Build history of the part. All positions in model axes, mm. A direction names the side the tool comes from. Give positions to 0.01 mm unless a question says otherwise; leave off trailing zeros. Write each loop counter-clockwise with the first axis right and the second up, starting at its lowest first coordinate (ties: lowest second). Pieces come first, ordered by that corner, then holes. Notation, with made-up numbers: (-6, 9.25) -> (7, 9.25) arc R18 ccw to (7, 32.25) -> close; hole circle Ø2 at (69.5, 9). An arc over 180 degrees is marked (long way). Put each result on its own line as item: value. Start each with the question number.
Item 1: Slice it at C-C, the plane y = 13. List the corners of the cut face in (x, z), plus the area to 3 significant figures.
Item 2: Tool access for faces 1 (the flat face through (38, 47, 0.5)), 2 (the flat face through (75.2, 12, 1)), 3 (the flat face through (-3, 35, 1)), 4 (the flat face through (75.2, 47, 1)), 5 (the flat face through (-4, 25, 1)): list every direction of +Z, -Z, +X, -X, +Y, -Y with a clear straight run to the whole face (end or side of a thin tool).
Item 3: Slice it at A-A, the plane y = 30. List the corners of the cut face in (x, z).
Item 4: Slice it at D-D, the plane y = 38.5. List the corners of the cut face in (x, z), plus the area to 3 significant figures.
Item 5: Flat gauge pins, fed straight in: pin 1 Ø3 at (x, y) = (36.5, 48.5) entering from +Z; pin 2 Ø0.6 at (x, z) = (78.5, 1) entering from +Y; pin 3 Ø6 at (x, y) = (18, 42.5) entering from -Z; pin 4 Ø2 at (x, y) = (82.2, 30) entering from +Z. Where does each tip first touch, or does it go through?
Item 6: Two-plate mould, pull along X, no slides. Class faces 6 (the flat face through (0, 47, 1)), 7 (the cylindrical face through (34.912, 8.784, 1.26)), 8 (the cylindrical face through (87.2, 30.1, 1)): pulls with the +X half, pulls with the -X half, needs draft (parallel to the pull), parting line crosses it, or undercut.
Item 7: Slice it at B-B, the plane x = 78. List the corners of the cut face in (y, z), plus the area to 3 significant figures.
Item 8: Drill centre lines: line 1 along Y through (x, z) = (37.6, 1.2); line 2 along Y through (x, z) = (-7, 1.5); line 3 along X through (y, z) = (13, 1). Where is each one in solid material? Low to high.
```python
from build123d import *

# Parameters (mm, degrees)
SKETCH2_W           = 75.2
SKETCH2_H           = 60
SKETCH2_R           = 1.65
BOSS_EXTRUDE1_DEPTH = 2
SKETCH3_R           = 5
CUT_EXTRUDE1_DEPTH  = 1.5


with BuildPart() as part:
    # Sketch2 → Boss-Extrude1 (new body)
    # profile 1 of 3: a face of its own
    with BuildSketch(Plane.XY):
        with Locations((37.6, 30)):
            Rectangle(SKETCH2_W, SKETCH2_H)
    # profile 2 of 3: a face of its own
    with BuildSketch(Plane.XY):
        with BuildLine():
            Line((0, 35), (-7, 35))
            ThreePointArc((-7, 35), (-12, 30), (-7, 25))
            Line((-7, 25), (0, 25))
            Line((0, 25), (0, 35))
        make_face()
        with Locations((-7, 30)):
            Circle(SKETCH2_R, mode=Mode.SUBTRACT)
    # profile 3 of 3: a face of its own
    with BuildSketch(Plane.XY):
        with BuildLine():
            Line((82.2, 25), (75.2, 25))
            Line((75.2, 25), (75.2, 35))
            Line((75.2, 35), (82.2, 35))
            ThreePointArc((82.2, 35), (87.2, 30), (82.2, 25))
        make_face()
        with Locations((82.2, 30)):
            Circle(SKETCH2_R, mode=Mode.SUBTRACT)
    extrude(amount=BOSS_EXTRUDE1_DEPTH)

    # Sketch3 → Cut-Extrude1 (cut)
    with BuildSketch(Plane.XY.offset(2)):
        with Locations((37.6, 47)):
            Circle(SKETCH3_R)
        with Locations(Location((37.6, 13, 0), (0, 0, 180))):
            Circle(SKETCH3_R)
    extrude(amount=-CUT_EXTRUDE1_DEPTH, mode=Mode.SUBTRACT)


solid = part.part
```
Values follow:
1. outline: (0, 0) -> (75.2, 0) -> (75.2, 2) -> (42.6, 2) -> (42.6, 0.5) -> (32.6, 0.5) -> (32.6, 2) -> (0, 2) -> close
1. area: 135 mm2
2. face 1: +Z
2. face 2: +Z, -Z, +X, -Y
2. face 3: +Z, -Z, -X, +Y
2. face 4: +Z, -Z, +X, +Y
2. face 5: +Z, -Z, -X, -Y
3. outline: (-12, 0) -> (-8.65, 0) -> (-8.65, 2) -> (-12, 2) -> close; (-5.35, 0) -> (80.55, 0) -> (80.55, 2) -> (-5.35, 2) -> close; (83.85, 0) -> (87.2, 0) -> (87.2, 2) -> (83.85, 2) -> close
4. outline: (0, 0) -> (75.2, 0) -> (75.2, 2) -> (0, 2) -> close
4. area: 150 mm2
5. pin 1: z = 0.5
5. pin 2: y = 35
5. pin 3: z = 0
5. pin 4: through
6. face 6: pulls with the -X half
6. face 7: undercut
6. face 8: pulls with the +X half
7. outline: (25, 0) -> (35, 0) -> (35, 2) -> (25, 2) -> close
7. area: 20.0 mm2
8. line 1: 0 to 8, 18 to 42, 52 to 60
8. line 2: 25 to 28.35, 31.65 to 35
8. line 3: 0 to 32.6, 42.6 to 75.2
